Input: part model. Units: mm. Frame: model coordinates. Coordinates: 2 decimals unless noted, no trailing zeros. Order: outer loops, then holes, each group sorted by start corner. A loop starts at its lowest first (then second) coordinate and runs counter-clockwise, first axis right, second up. Notation, with made-up numbers: (80.25, 60.5) -> (122.25, 60.5) arc R26 ccw to (122.25, 83.5) -> close; hole circle Ø2 at (43, 21.5). An arc over 180 degrees is marked (long way). Use one line per item in the form item = value. Start each with the question number.
1) Pin query (flat end, axial travel): pin 1 (3 mm diameter, centred on x = 53, y = -2, fed in from -Z); pin 2 (8 mm diameter, centred on x = 134.5, z = 55.5, fed in from -Y) (3 decimals); pin 3 (3 mm diameter, centred on x = 169, y = 9, fed in from -Z). Return the tip coordinate at first contact, or that it passes through.
2) Section query A-A on z = 38.1. Output: boundary loops of the cut face in (x, y).
3) Section query D-D on x = 175.5. Output: boundary loops of the cut face in (y, z) (3 decimals).
4) Section query B-B on x = 62.5. Output: boundary loops of the cut face in (y, z) (3 decimals), then the cut area to 3 significant figures.
5) Section query C-C on y = 23. Output: boundary loops of the cut face in (x, z).
6) Ray query, line 1 along Z through (x, y) = (257.5, 13); line 2 along Z through (x, y) = (221, 5.5); line 3 along Y through (x, z) = (70.5, 37). Return the intervals inside material, ascending.
7) Draft query along Z for faces 1 (the flat face through (21, -3, 6.35)), 2 (the flat face through (308, 38.1, 57)). Return one class per face: pulls with the +Z half, pulls with the -Z half, needs draft (parallel to the pull), parting line crosses it, or undercut.
from build123d import *

# Parameters (mm, degrees)
F1_DEPTH  = 304.8
F2_W      = 25.4
F2_H      = 63.5
F3_DEPTH  = 6.35
F4_W      = 25.4
F4_H      = 63.5
F5_DEPTH  = 6.35
F6_W      = 304.8
F6_H      = 76.2
F6_W_2    = 292.099996
F6_H_2    = 63.499996
F7_DEPTH  = 6.35
F9_DEPTH  = 6.35
F10_R     = 12.18433
F10_R_2   = 12.378685
F10_R_3   = 12.666462
F10_R_4   = 13.33955
F10_R_5   = 12.965917
F10_R_6   = 12.911659
F10_R_7   = 12.980347
F10_R_8   = 12.853529
F10_R_9   = 12.732802
F10_R_10  = 12.333231
F10_R_11  = 12.306635
F10_R_12  = 13.272723
F10_R_13  = 12.908035
F10_R_14  = 12.255033
F10_R_15  = 12.911662
F10_R_16  = 12.143618
F11_DEPTH = 3.175


with BuildPart() as f1:
    # F0 (on Right) → F1 (new body)
    with BuildSketch(Plane.YZ):
        with BuildLine():
            Line((0, 76.2), (0, 0))
            ThreePointArc((0, 0), (45.114366, 38.1), (0, 76.2))
        make_face()
    extrude(amount=F1_DEPTH)

    # F2 (on face) → F3 (join)
    with BuildSketch(Plane(origin=(0, 0, 0), x_dir=(0, -1, 0), z_dir=(-1, 0, 0))):
        with Locations((-25.4, 57.15)):
            Rectangle(F2_W, F2_H)
    extrude(amount=F3_DEPTH)

    # F4 (on face) → F5 (join)
    with BuildSketch(Plane.YZ.offset(304.8)):
        with Locations((25.4, 57.15)):
            Rectangle(F4_W, F4_H)
    extrude(amount=F5_DEPTH)

    # F6 (on face) → F7 (join)
    with BuildSketch(Plane.XZ):
        with Locations((152.4, 38.1)):
            Rectangle(F6_W, F6_H)
        with Locations((152.4, 38.1)):
            Rectangle(F6_W_2, F6_H_2, mode=Mode.SUBTRACT)
    extrude(amount=F7_DEPTH)

    # F8 (on face) → F9 (join)
    with BuildSketch(Plane.XZ):
        Polygon((298.449998, 34.925), (298.449998, 41.275), (266.241582, 41.275), (266.241582, 69.849998), (259.891582, 69.849998), (259.891582, 41.275), (229.023391, 41.275), (229.023391, 69.849998), (222.673391, 69.849998), (222.673391, 41.275), (192.373246, 41.275), (192.373246, 69.849998), (186.023246, 69.849998), (186.023246, 41.275), (155.575, 41.275), (155.575, 69.849998), (149.225, 69.849998), (149.225, 41.275), (116.587477, 41.275), (116.587477, 69.849998), (110.237477, 69.849998), (110.237477, 41.275), (79.624019, 41.275), (79.624019, 69.849998), (73.274019, 69.849998), (73.274019, 41.275), (41.912001, 41.275), (41.912001, 69.849998), (35.562001, 69.849998), (35.562001, 41.275), (6.350002, 41.275), (6.350002, 34.925), (35.562001, 34.925), (35.562001, 6.350002), (41.912001, 6.350002), (41.912001, 34.925), (73.274019, 34.925), (73.274019, 6.350002), (79.624019, 6.350002), (79.624019, 34.925), (110.237477, 34.925), (110.237477, 6.350002), (116.587477, 6.350002), (116.587477, 34.925), (149.225, 34.925), (149.225, 6.350002), (155.575, 6.350002), (155.575, 34.925), (186.023246, 34.925), (186.023246, 6.350002), (192.373246, 6.350002), (192.373246, 34.925), (222.673391, 34.925), (222.673391, 6.350002), (229.023391, 6.350002), (229.023391, 34.925), (259.891582, 34.925), (259.891582, 6.350002), (266.241582, 6.350002), (266.241582, 34.925), align=None)
    extrude(amount=F9_DEPTH)

    # F10 (on face) → F11 (join)
    with BuildSketch(Plane.XZ):
        with Locations((20.775795, 55.44908)):
            Circle(F10_R)
        with Locations((56.877859, 55.44908)):
            Circle(F10_R_2)
        with Locations((21.387694, 21.182716)):
            Circle(F10_R_3)
        with Locations((56.877859, 21.182716)):
            Circle(F10_R_4)
        with Locations((94.509669, 56.672879)):
            Circle(F10_R_5)
        with Locations((95.12157, 20.876767)):
            Circle(F10_R_6)
        with Locations((132.447436, 56.060981)):
            Circle(F10_R_7)
        with Locations((132.141486, 20.876767)):
            Circle(F10_R_8)
        with Locations((170.691147, 56.366932)):
            Circle(F10_R_9)
        with Locations((170.079246, 21.182716)):
            Circle(F10_R_10)
        with Locations((207.405105, 55.143133)):
            Circle(F10_R_11)
        with Locations((206.793204, 20.570816)):
            Circle(F10_R_12)
        with Locations((244.217366, 55.595852)):
            Circle(F10_R_13)
        with Locations((244.217366, 21.182716)):
            Circle(F10_R_14)
        with Locations((282.155126, 55.901799)):
            Circle(F10_R_15)
        with Locations((282.461077, 21.182716)):
            Circle(F10_R_16)
    extrude(amount=F11_DEPTH)


solid = f1.part
Answers below:
q1.pin_1 = 0
q1.pin_2 = -3.175
q1.pin_3 = -0.53
q2.outline = (-6.35, 12.7) -> (0, 12.7) -> (0, -6.35) -> (304.8, -6.35) -> (304.8, 12.7) -> (311.15, 12.7) -> (311.15, 38.1) -> (304.8, 38.1) -> (304.8, 45.11) -> (0, 45.11) -> (0, 38.1) -> (-6.35, 38.1) -> close
q3.outline = (-6.35, 0) -> (0, 0) arc R38.645 ccw (long way) to (0, 76.2) -> (-6.35, 76.2) -> (-6.35, 69.85) -> (0, 69.85) -> (0, 68.157) -> (-3.175, 68.157) -> (-3.175, 44.577) -> (0, 44.577) -> (0, 41.275) -> (-6.35, 41.275) -> (-6.35, 34.925) -> (0, 34.925) -> (0, 32.261) -> (-3.175, 32.261) -> (-3.175, 10.105) -> (0, 10.105) -> (0, 6.35) -> (-6.35, 6.35) -> close
q4.outline = (-6.35, 0) -> (0, 0) arc R38.645 ccw (long way) to (0, 76.2) -> (-6.35, 76.2) -> (-6.35, 69.85) -> (0, 69.85) -> (0, 66.477) -> (-3.175, 66.477) -> (-3.175, 44.421) -> (0, 44.421) -> (0, 41.275) -> (-6.35, 41.275) -> (-6.35, 34.925) -> (0, 34.925) -> (0, 33.28) -> (-3.175, 33.28) -> (-3.175, 9.086) -> (0, 9.086) -> (0, 6.35) -> (-6.35, 6.35) -> close
q4.area = 3,110 mm^2
q5.outline = (-6.35, 25.4) -> (0, 25.4) -> (0, 3.17) -> (304.8, 3.17) -> (304.8, 25.4) -> (311.15, 25.4) -> (311.15, 88.9) -> (304.8, 88.9) -> (304.8, 73.03) -> (0, 73.03) -> (0, 88.9) -> (-6.35, 88.9) -> close
q6.line_1 = 0.01 to 76.19
q6.line_2 = -0.53 to 76.73
q6.line_3 = -6.35 to 45.1
q7.face_1 = undercut
q7.face_2 = needs draft
